For this review, take the finished solid that the model builds, in its own axes (mm). Face numbers are marked on the shaded views. A direction names the side the tool comes from. Round coordinates to 2 decimals unless told otherwise and drop trailing zeros. Write each loop counter-clockwise with the first axis right and the second up, starting at its lowest first coordinate (ties: lowest second). Pieces come first, ordered by that corner, then holes. Notation, with made-up numbers: (-15.75, 62.25) - (19.25, 62.25) arc R27 ccw to (19.25, 98.25) - close; hole circle Ø10 at (25, -27.75). An arc over 180 degrees is marked (long way). Answer in a Markdown table with one row per item. Add a question column.
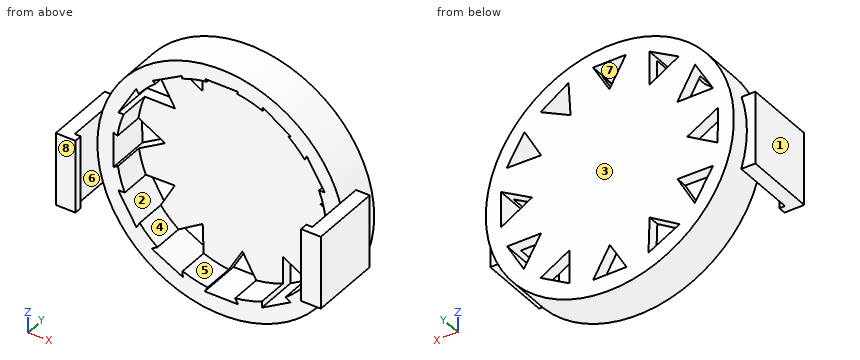
Autodesk Inventor part; units mm, degrees
ref_plane "YZ Plane" through (0, 0, 0) normal (1, 0, 0) x (0, 1, 0)
ref_plane "XZ Plane" through (0, 0, 0) normal (0, 1, 0) x (-1, 0, 0)
ref_plane "XY Plane" through (0, 0, 0) normal (0, 0, 1) x (1, 0, 0)
sketch "Sketch1" plane through (0, 0, 0) normal (0, 1, 0) x (-1, 0, 0)
  circle A0 centre (0, 0) radius 22
  arc A1 (-13.7238, -17.1947) -> (13.7238, -17.1947) centre (0, 0) ccw
  dimension "d0" = 44
  dimension "d11" = 13.7238
ref_plane "Work Plane10" through (0, 7, 0) normal (0, 1, 0) x (1, 0, 0)
sketch "Sketch5" plane through (0, 7, 0) normal (0, 1, 0) x (1, 0, 0)
  circle A0 centre (0, 0) radius 20
  dimension "d8" = 40
ref_plane "Work Plane9" through (0, 0, 0) normal (0, -1, 0) x (1, 0, 0)
sketch "Sketch8" plane through (0, 0, 0) normal (0, -1, 0) x (1, 0, 0)
  arc A0 (-11.5874, -18.7011) -> (11.5874, -18.7011) centre (0, 0) ccw
  line L0 (-15.0453, -16.0511) -> (-15.0453, -22.0257)
  line L1 (15.0453, -16.0511) -> (15.0453, -22.0257)
  arc A1 (-15.0453, -16.0511) -> (15.0453, -16.0511) centre (0, 0) ccw
  arc A2 (-15.0453, -22.0257) -> (-13.0453, -24.0257) centre (-13.0453, -22.0257) ccw
  arc A3 (13.0453, -24.0257) -> (15.0453, -22.0257) centre (13.0453, -22.0257) ccw
  line L2 (-15.0451, -16.0514) -> (-15.0451, -22.026)
  arc A4 (-15.0451, -22.026) -> (-13.0451, -24.026) centre (-13.0451, -22.026) ccw
  arc A5 (13.0456, -24.026) -> (15.0456, -22.026) centre (13.0456, -22.026) ccw
  line L3 (15.0456, -16.0514) -> (15.0456, -22.026)
  arc A6 (-15.0451, -16.0514) -> (15.0456, -16.0514) centre (0.0003, -0.0002) ccw
  arc A7 (13.0456, -24.026) -> (-13.0451, -24.026) centre (0.0003, -66.8475) ccw
  point P0 (0, 0)
  point P1 (0, 0)
ref_plane "Work Plane8" through (0, 0, 0) normal (0, -1, 0) x (1, 0, 0)
sketch "Sketch11" plane through (0, 0, 0) normal (0, -1, 0) x (1, 0, 0)
  arc A0 (11.5874, 18.7011) -> (-11.5874, 18.7011) centre (0, 0) ccw
  line L0 (-15.0453, 16.0511) -> (-15.0453, 22.0257)
  line L1 (15.0453, 16.0511) -> (15.0453, 22.0257)
  arc A1 (15.0453, 16.0511) -> (-15.0453, 16.0511) centre (0, 0) ccw
  arc A2 (-13.0453, 24.0257) -> (-15.0453, 22.0257) centre (-13.0453, 22.0257) ccw
  arc A3 (15.0453, 22.0257) -> (13.0453, 24.0257) centre (13.0453, 22.0257) ccw
  line L2 (-15.0451, 16.0514) -> (-15.0451, 22.026)
  arc A4 (-13.0451, 24.026) -> (-15.0451, 22.026) centre (-13.0451, 22.026) ccw
  arc A5 (15.0456, 22.026) -> (13.0456, 24.026) centre (13.0456, 22.026) ccw
  line L3 (15.0456, 16.0514) -> (15.0456, 22.026)
  arc A6 (15.0456, 16.0514) -> (-15.0451, 16.0514) centre (0.0003, 0.0002) ccw
  arc A7 (-13.0451, 24.026) -> (13.0456, 24.026) centre (0.0003, 66.8475) ccw
  point P0 (0, 0)
  dimension "d27" = 2
  dimension "d28" = 2
ref_plane "Work Plane5" through (14.0456, 0, 22.026) normal (1, 0, 0) x (0, 0, -1)
sketch "Sketch14" plane through (14.0456, 0, 22.026) normal (1, 0, 0) x (0, 0, -1)
  line L0 (0, 0) -> (0, 7)
  circle A0 centre (0, 3.5) radius 0.9
  point P0 (22.026, 0)
  dimension "d38" = 1.8
ref_plane "Work Plane6" through (14.0456, 0, 22.026) normal (1, 0, 0) x (0, 0, -1)
sketch "Sketch15" plane through (14.0456, 0, 22.026) normal (1, 0, 0) x (0, 0, -1)
  line L0 (44.1089, 7) -> (44.1089, 0)
  circle A0 centre (44.1089, 3.5) radius 0.9
  point P0 (22.026, 0)
  dimension "d41" = 1.8
ref_plane "Work Plane7" through (0, 7, 0) normal (0, 1, 0) x (1, 0, 0)
sketch "Sketch16" plane through (0, 7, 0) normal (0, 1, 0) x (1, 0, 0)
  circle A0 centre (0, 0) radius 22
  circle A1 centre (0, -0.3745) radius 18.6
  dimension "d44" = 37.2
extrude "Extrusion13" add sketch "Sketch16" along normal blind 7.5
ref_plane "Work Plane3" through (22, 0, 0) normal (1, 0, 0) x (0, 1, 0)
sketch "Sketch17" plane through (22, 0, 0) normal (1, 0, 0) x (0, 1, 0)
  line L0 (7, -18.2255) -> (7, 18.9745)
  line L1 (11.1125, 6.35) -> (7, 6.35)
  line L2 (7, 6.35) -> (7, -6.5465)
  line L3 (7, -6.5465) -> (11.1125, -6.5465)
  line L4 (11.1125, -6.5465) -> (11.1125, 6.35)
extrude "Extrusion14" add sketch "Sketch17" along normal mid plane 3
ref_plane "Work Plane12" through (21.0034, 7, -6.5465) normal (0, -1, 0) x (1, 0, 0)
sketch "Sketch18" plane through (21.0034, 7, -6.5465) normal (0, -1, 0) x (1, 0, 0)
  arc A0 (-35.8073, -9.7276) -> (-35.8073, 22.8206) centre (-21.0034, 6.5465) ccw
  line L0 (0, 0) -> (2.4966, 0)
  line L1 (0, 0) -> (2.4966, 0)
  line L2 (2.4966, 12.8965) -> (0.0602, 12.8965)
  line L3 (2.4966, 0) -> (2.4966, 12.8965)
  line L4 (2.4966, 12.8965) -> (0.0602, 12.8965)
  arc A1 (0, 0) -> (0.0602, 12.8965) centre (-21.0034, 6.5465) ccw
extrude "Extrusion15" add sketch "Sketch18" along normal blind 8.65
ref_plane "Work Plane4" through (-22, 0, 0) normal (-1, 0, 0) x (0, -1, 0)
sketch "Sketch19" plane through (-22, 0, 0) normal (-1, 0, 0) x (0, -1, 0)
  line L0 (-11.1125, -6.5465) -> (-11.1125, 6.35)
  line L1 (-7, -20) -> (-7, 20)
  line L2 (-11.1125, -6.5465) -> (-7, -6.5465)
  line L3 (-7, -6.5465) -> (-7, 6.35)
  line L4 (-7, 6.35) -> (-11.1125, 6.35)
  line L5 (-11.1125, 6.35) -> (-11.1125, -6.5465)
  point P0 (0, 0)
extrude "Extrusion16" add sketch "Sketch19" along normal mid plane 3
sketch "Sketch20" plane through (-23.5, 7, -6.5465) normal (0, -1, 0) x (1, 0, 0)
  line L0 (0, 0) -> (2.4966, 0)
  line L1 (2.4966, 0) -> (0, 0)
  line L2 (0, 12.8965) -> (0, 0)
  line L3 (0, 0) -> (0, 12.8965)
  arc A0 (2.4363, 12.8965) -> (2.4966, 0) centre (23.5, 6.5465) ccw
  line L4 (0, 12.8965) -> (2.4363, 12.8965)
  point P0 (3, 0)
extrude "Extrusion17" add sketch "Sketch20" along normal blind 8.65
sketch "Sketch21" plane through (-23.5, 0, 0) normal (-1, 0, 0) x (0, 0, 1)
  line L0 (-6.5465, 11.1125) -> (-6.5465, -1.65)
  line L1 (6.35, -1.65) -> (-6.5465, -1.65)
  line L2 (-6.5465, -1.65) -> (-6.5465, -0.292)
  line L3 (-6.5465, -0.292) -> (6.35, -0.292)
  line L4 (6.35, -0.292) -> (6.35, -1.65)
  point P0 (6.35, 0)
extrude "Extrusion18" add sketch "Sketch21" against normal blind 3.5
sketch "Sketch22" plane through (23.5, 0, 0) normal (1, 0, 0) x (0, 0, -1)
  line L0 (-6.35, -0.292) -> (6.5465, -0.292)
  line L1 (-6.35, -1.65) -> (6.5465, -1.65)
  line L2 (6.5465, -0.292) -> (-6.35, -0.292)
  line L3 (-6.35, -0.292) -> (-6.35, -1.65)
  line L4 (-6.35, -1.65) -> (6.5465, -1.65)
  line L5 (6.5465, -1.65) -> (6.5465, -0.292)
  point P0 (0, 0)
extrude "Extrusion19" add sketch "Sketch22" against normal blind 3.5
ref_plane "Work Plane11" through (0, 14.5, 0) normal (0, 1, 0) x (1, 0, 0)
sketch "Sketch23" plane through (0, 14.5, 0) normal (0, 1, 0) x (1, 0, 0)
  circle A0 centre (0, 0) radius 20
extrude "Extrusion20" add sketch "Sketch23" against normal blind 2
sketch "Sketch24" plane through (0, 14.5, 0) normal (0, 1, 0) x (1, 0, 0)
  line L0 (2.958, 18.9599) -> (-0.0041, 13.8437)
  line L1 (-0.0041, 13.8437) -> (-2.9538, 18.9671)
  line L2 (-2.9538, 18.9671) -> (2.958, 18.9599)
  line L3 (12.2922, 14.893) -> (7.1379, 11.9475)
  line L4 (7.1379, 11.9475) -> (7.1641, 17.884)
  line L5 (7.1641, 17.884) -> (12.2922, 14.893)
  line L6 (18.2225, 6.8835) -> (12.2004, 6.928)
  line L7 (12.2004, 6.928) -> (15.25, 12.1211)
  line L8 (15.25, 12.1211) -> (18.2225, 6.8835)
  line L9 (19.2871, 3.0371) -> (19.2959, -3.302)
  line L10 (19.2959, -3.302) -> (13.8017, -0.1401)
  line L11 (13.8017, -0.1401) -> (19.2871, 3.0371)
  line L12 (18.3039, -7.2042) -> (15.1393, -12.4356)
  line L13 (15.1393, -12.4356) -> (12.1912, -7.0793)
  line L14 (12.1912, -7.0793) -> (18.3039, -7.2042)
  line L15 (12.2922, -14.8615) -> (7.3345, -18.1476)
  line L16 (7.3345, -18.1476) -> (6.9675, -12.2111)
  line L17 (6.9675, -12.2111) -> (12.2922, -14.8615)
  line L18 (0.0704, -14.1349) -> (2.9797, -19.1738)
  line L19 (2.9797, -19.1738) -> (-2.8388, -19.1738)
  line L20 (-2.8388, -19.1738) -> (0.0704, -14.1349)
  line L21 (-7.0607, -12.1336) -> (-7.0172, -18.0963)
  line L22 (-7.0172, -18.0963) -> (-12.2028, -15.1526)
  line L23 (-12.2028, -15.1526) -> (-7.0607, -12.1336)
  line L24 (-11.9565, -7.0793) -> (-15.118, -12.5587)
  line L25 (-15.118, -12.5587) -> (-18.2826, -7.0811)
  line L26 (-18.2826, -7.0811) -> (-11.9565, -7.0793)
  line L27 (-13.7277, -0.1539) -> (-19.1828, -3.2194)
  line L28 (-19.1828, -3.2194) -> (-19.11, 3.0377)
  line L29 (-19.11, 3.0377) -> (-13.7277, -0.1539)
  line L30 (-11.9985, 6.7691) -> (-18.3039, 6.8788)
  line L31 (-18.3039, 6.8788) -> (-15.0562, 12.2846)
  line L32 (-15.0562, 12.2846) -> (-11.9985, 6.7691)
  line L33 (-7.0607, 11.7045) -> (-12.3714, 15.0155)
  line L34 (-12.3714, 15.0155) -> (-6.8486, 17.9592)
  line L35 (-6.8486, 17.9592) -> (-7.0607, 11.7045)
  point P0 (0, 0)
  point P1 (0, 17.2569)
  point P2 (8.8647, 14.9082)
  point P3 (15.2243, 8.6442)
  point P4 (17.4616, -0.135)
  point P5 (15.2115, -8.9064)
  point P6 (8.8647, -15.0734)
  point P7 (0.0704, -17.4941)
  point P8 (-8.7603, -15.1275)
  point P9 (-15.119, -8.9064)
  point P10 (-17.3402, -0.1119)
  point P11 (-15.1196, 8.6442)
  point P12 (-8.7603, 14.893)
extrude "Extrusion21" cut sketch "Sketch24" against normal blind 8
properties part number "watchBodyOneTopV1.1"
Q1. Tool access review of the marked faces 5, 6, 7 and 8: name each direction out of +Z, -Z, +X, -X, +Y, -Y from which nothing blocks a thin tool from reaching the whole face with its end or side.
Q2. Add section C-C on z = -16. State the section outline as (x, y) points, then the cut area to 3 significant figures.
Q3. Add section B-B on x = 10.5. State the section outline as (y, z) points.
Q4. Insertion check: pin 1 Ø4 at (x, y) = (21, 3.5) entering from -Z; pin 2 Ø1.5 at (x, z) = (-18, 1.5) entering from +Y; pin 3 Ø3 at (x, y) = (22.5, 5) entering from +Z; pin 4 Ø3 at (y, z) = (11.5, 11.5) entering from +X. Each pin has a flat end and moves straight along its axis. Give the tip position at first contact, or say it passes through.
Q5. Draft analysis for pull direction X (two halves, no side actions). For the marked faces 1, 2, 3 and 4, state which applies: released by +X, released by -X, zero draft, split by the parting line, or undercut.
Q6. Add section A-A on y = 5.5. State the section outline as (x, z) points, then the cut area to 3 significant figures.
Q7. Add section D-D on x = -4.5. State the section outline as (y, z) points, then the cut area to 3 significant figures.
Q8. To check wall thickness, follow probe 1 along Z at (x, y) = (9.5, 12.75); probe 2 along Y at (x, z) = (-20.5, 6); probe 3 along X at (y, z) = (5, 0). State the ranges of each line that lie inside material, in increasing order.
Answer sheet:
| question | item | result |
|---|---|---|
| 1 | face 5 | -Y |
| 1 | face 6 | none |
| 1 | face 7 | +Y, -Y |
| 1 | face 8 | +Z, -Z, +X, -X, -Y |
| 2 | outline | (-15.1, 7) - (-10.52, 7) - (-10.52, 14.5) - (-15.1, 14.5) - close; (-6.92, 12.5) - (-1.25, 12.5) - (-1.25, 14.5) - (-6.92, 14.5) - close; (1.24, 12.5) - (7.16, 12.5) - (7.16, 14.5) - (1.24, 14.5) - close; (10.39, 7) - (15.1, 7) - (15.1, 14.5) - (10.39, 14.5) - close |
| 2 | area | 92.8 mm² |
| 3 | outline | (7, -19.33) - (14.5, -19.33) - (14.5, -15.94) - (7, -15.94) - close; (7, 16.05) - (14.5, 16.05) - (14.5, 19.33) - (7, 19.33) - close; (12.5, -13.87) - (14.5, -13.87) - (14.5, 13.97) - (12.5, 13.97) - close |
| 4 | pin 1 | stops at z = -6.55 |
| 4 | pin 2 | passes through |
| 4 | pin 3 | stops at z = 6.35 |
| 4 | pin 4 | stops at x = 19.6 |
| 5 | face 1 | released by -X |
| 5 | face 2 | undercut |
| 5 | face 3 | zero draft |
| 5 | face 4 | undercut |
| 6 | outline | (-23.5, -6.55) - (-21, -6.55) arc R22 cw to (-21.06, 6.35) - (-23.5, 6.35) - close; (21, -6.55) - (23.5, -6.55) - (23.5, 6.35) - (21.06, 6.35) arc R22 cw to start |
| 6 | area | 46.9 mm² |
| 7 | outline | (7, -21.53) - (14.5, -21.53) - (14.5, 21.53) - (7, 21.53) - (7, 18.42) - (12.5, 18.42) - (12.5, -17.67) - (7, -17.67) - close |
| 7 | area | 125 mm² |
| 8 | probe 1 | z = -19.84 to -16.52, -13.3 to 13.47, 16.71 to 19.84 |
| 8 | probe 2 | y = -1.65 to -0.29, 7 to 14.5 |
| 8 | probe 3 | x = -23.5 to -22, 22 to 23.5 |
